```python
from build123d import *

# Parameters (mm, degrees)
SKETCH2_W           = 50
SKETCH2_H           = 44
BOSS_EXTRUDE2_DEPTH = 76
CUT_EXTRUDE1_DEPTH  = 76
CUT_EXTRUDE2_DEPTH  = 76
SKETCH14_R          = 4
CUT_EXTRUDE3_DEPTH  = 20


with BuildPart() as part:
    # Sketch2 → Boss-Extrude2 (new body)
    with BuildSketch(Plane(origin=(0, 0, 0), x_dir=(1, 0, 0), z_dir=(0, 1, 0))):
        with Locations((-25, 22)):
            Rectangle(SKETCH2_W, SKETCH2_H)
    extrude(amount=BOSS_EXTRUDE2_DEPTH)

    # Sketch3 → Cut-Extrude1 (cut)
    with BuildSketch(Plane.XY):
        Polygon((-50, 76), (0, 47.132486541), (0, 76), align=None)
    extrude(amount=-CUT_EXTRUDE1_DEPTH, mode=Mode.SUBTRACT)

    # Sketch10 → Cut-Extrude2 (cut)
    with BuildSketch(Plane(origin=(23.262165395, 15.547974941, -11.734548971), x_dir=(0.3215470193165547, 0.21491571888839583, 0.9221815158326062), z_dir=(-0.7666944497450301, -0.5124435274969221, 0.38675735527159244))):
        Polygon((-4.625392025, 39.185578124), (-34.988178006, 63.006463096), (-34.988178006, 21.61619524), align=None)
    extrude(amount=-CUT_EXTRUDE2_DEPTH, mode=Mode.SUBTRACT)

    # Sketch14 → Cut-Extrude3 (cut)
    with BuildSketch(Plane(origin=(23.262165395, 15.547974941, -11.734548971), x_dir=(0.3215470193165547, 0.21491571888839583, 0.9221815158326062), z_dir=(-0.7666944497450301, -0.5124435274969221, 0.38675735527159244))):
        with Locations(Location((-22.531650424, 40.498325306, 0), (0, 0, 270))):
            Circle(SKETCH14_R)
    extrude(amount=CUT_EXTRUDE3_DEPTH, mode=Mode.SUBTRACT)


solid = part.part
```
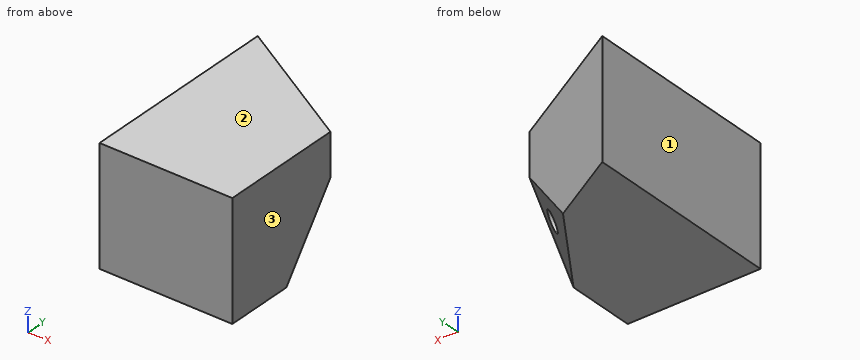
Work out the finished part from the listing and answer in its coordinate system (mm). Face numbers are marked on the shaded views. Round coordinates to 2 decimals unless told otherwise and drop trailing zeros. Loops run counter-clockwise (first coordinate to the right, second up) from the corner with the lowest first, then second, coordinate; pieces in that order, holes last. Notation, with made-up numbers: M 14,44.5 L 32,44.5 A28 ccw 32,77.5 Z; hole C 62.25,-34 d3. An arc over 180 degrees is marked long. One line per question, with ' | ' between items.
Q1. Each of these flat-tipped pins is pushed along its axis until it touches: pin 1 Ø6 at (x, z) = (-24, -39) entering from +Y; pin 2 Ø4 at (x, z) = (-31.5, -30.5) entering from +Y. Where does it stop, or does it pass through?
Conclusion:
pin 1: stops at y = 62.72 | pin 2: stops at y = 66.47
Q2. Find section B-B, the plane y = 63. Give the vertices of the cut face in (x, z).
Conclusion:
outline: M -50,-44 L -27.48,-44 L -27.48,0 L -50,0 Z
Q3. Consider line 1 along X through (y, z) = (38.5, -29); line 2 along Z through (x, y) = (-17, 39.5); line 3 along Y through (x, z) = (-40, -12). Determine where each line is inside the solid, lowest interval first. Write a range as from..to.
Conclusion:
line 1: x = -50..-20.74, -8.49..-0.79 | line 2: z = -44..-31.59, -23.83..0 | line 3: y = 0..70.23
Q4. The mould has two halves that part along X. Classify the marked faces 1, 2 and 3: +X half, -X half, draft (parallel to the pull), parting line (faces both ways), or undercut.
Conclusion:
face 1: -X half | face 2: draft | face 3: +X half
Q5. Find section C-C, the plane x = -38. Give the vertices of the cut face in (y, z).
Conclusion:
outline: M 0,-44 L 69.07,-44 L 69.07,0 L 0,0 Z
Q6. Find section D-D, the plane z = -18.5. Give the vertices of the cut face in (x, y).
Conclusion:
outline: M -50,0 L 0,0 L 0,45.25 L -2.05,48.32 L -50,76 Z
Q7. Find section A-A, the plane z = -39.5. Give the vertices of the cut face in (x, y).
Conclusion:
outline: M -50,0 L 0,0 L 0,29.4 L -19.3,58.28 L -50,76 Z
